The listing builds one solid part. Answer for the finished solid, in the listing's coordinates (mm). Give positions to 0.01 mm unless a question says otherwise; leave off trailing zeros. Order: outer loops, then holes, each group sorted by start corner. A loop starts at its lowest first (then second) coordinate and runs counter-clockwise, first axis right, second up. Notation, with made-up numbers: (89, 63) -> (114, 63) arc R23 cw to (114, 101) -> close; hole circle Ø4 at (27, 68.5). An arc over 180 degrees is marked (long way). Answer as a JSON object with one key per item and string values. Group by question number.
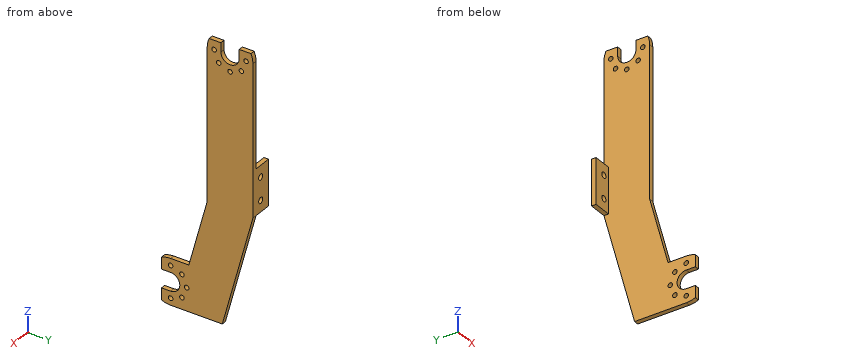
Autodesk Inventor part; units mm, degrees
ref_plane "YZ Plane" through (0, 0, 0) normal (1, 0, 0) x (0, 1, 0)
ref_plane "XZ Plane" through (0, 0, 0) normal (0, 1, 0) x (-1, 0, 0)
ref_plane "XY Plane" through (0, 0, 0) normal (0, 0, 1) x (1, 0, 0)
sketch "スケッチ1" plane through (0, 0, 0) normal (1, 0, 0) x (0, 1, 0)
  line L0 (-20, 60) -> (20, 60)
  line L1 (20, 60) -> (20, -60)
  line L2 (20, -60) -> (-20, -60)
  line L3 (-20, -60) -> (-20, 60)
  point P0 (0, 0)
  dimension "d0" = 120
  dimension "d2" = 40
  dimension "d3" = 20
  dimension "d4" = 60
extrude "押し出し1" add sketch "スケッチ1" along normal blind 2
sketch "スケッチ3" plane through (0, 0, 0) normal (-1, 0, 0) x (0, 0, 1)
  line L0 (60, -20) -> (60, 20)
  line L1 (60, 20) -> (-60, 20)
  line L2 (-60, 20) -> (-60, -20)
  line L3 (-60, -20) -> (60, -20)
  line L4 (-40, -20) -> (-40, -8.0385)
  line L5 (-40, -8.0385) -> (-10, 0)
  line L6 (-10, 0) -> (60, 0)
  line L7 (60, 0) -> (60, 20)
  line L8 (-60, 6.6025) -> (-10, 20)
  point P0 (0, 0)
  dimension "d11" = 20
  dimension "d12" = 15
  dimension "d13" = 15
  dimension "d14" = 20
  dimension "d15" = 120
  dimension "d17" = 70
  dimension "d18" = 70
extrude "押し出し3" cut sketch "スケッチ3" against normal blind 20 contours L6 L5 L4 L3 L2 L8 L1 L0 keep common part
sketch "スケッチ6" plane through (0, 0, 0) normal (-1, 0, 0) x (0, 0, 1)
  line L0 (-40, -8.0385) -> (-40, -20)
  line L1 (-10, 0) -> (-40, -8.0385)
  line L2 (60, 0) -> (-10, 0)
  line L3 (60, 0) -> (60, 20)
  line L4 (60, 20) -> (-10, 20)
  line L5 (-60, 6.6025) -> (-10, 20)
  line L6 (-60, 6.6025) -> (-60, -20)
  line L7 (-60, -20) -> (-40, -20)
  arc A0 (-46, -16) -> (-54, -16) centre (-50, -16) ccw
  arc A1 (56, 14) -> (56, 6) centre (56, 10) ccw
  line L8 (-54, -16) -> (-54, -20)
  line L9 (-46, -16) -> (-46, -20)
  line L10 (56, 14) -> (60, 14)
  line L11 (56, 6) -> (60, 6)
  arc A2 (-40.8348, -20) -> (-40, -16) centre (-50, -16) ccw
  arc A3 (-60, -16) -> (-59.1652, -20) centre (-50, -16) ccw
  arc A4 (56, 0) -> (60, 0.8348) centre (56, 10) ccw
  arc A5 (60, 19.1652) -> (56, 20) centre (56, 10) ccw
  point P0 (0, 0)
  dimension "d39" = 8
  dimension "d40" = 4
  dimension "d41" = 4
  dimension "d42" = 10
  dimension "d43" = 10
extrude "押し出し6" cut sketch "スケッチ6" against normal blind 11 contours L0 A2 L7 L9 A0 L8 A3 L6 L5 L4 A5 L3 L10 A1 L11 A4 L2 L1 keep common part
sketch "スケッチ7" plane through (0, 0, 0) normal (-1, 0, 0) x (0, 0, 1)
  arc A0 (60, 19.1652) -> (56, 20) centre (56, 10) ccw
  arc A1 (-60, -16) -> (-59.1652, -20) centre (-50, -16) ccw
  line L0 (-59.1652, -20) -> (-54, -20)
  line L1 (60, 0.8348) -> (60, 6)
  circle A2 centre (56, 3) radius 1
  circle A3 centre (-57, -16) radius 1
  point P0 (0, 0)
  dimension "d46" = 2
  dimension "d48" = 7
  dimension "d49" = 4
  dimension "d50" = 4
  dimension "d51" = 7
hole "穴1" at (0, -16, -57) at (0, 3, 56) direction (1, 0, 0) diameter 2 end through all
pattern_circular "円形状パターン1" count 5 over 180 about axis through (0, -16, -50) along (1, 0, 0) of "穴1"
pattern_circular "円形状パターン2" count 5 over 180 about axis through (0, 10, 56) along (1, 0, 0) of "穴1"
sketch "スケッチ9" plane through (0, 0, 0) normal (-1, 0, 0) x (0, 0, 1)
  line L0 (56, 20) -> (-10, 20)
  line L1 (60, 14) -> (60, 19.1652)
  line L2 (10, 20) -> (-10, 20)
  line L3 (-10, 20) -> (-10, 18)
  line L4 (-10, 18) -> (10, 18)
  line L5 (10, 18) -> (10, 20)
  point P0 (0, 0)
  dimension "d85" = 2
  dimension "d87" = 20
  dimension "d88" = 50
extrude "押し出し8" add sketch "スケッチ9" along normal blind 8
sketch "スケッチ10" plane through (0, 20, 56) normal (0, 1, 0) x (1, 0, 0)
  line L0 (0, 66) -> (-8, 66)
  line L1 (-8, 46) -> (-8, 66)
  circle A0 centre (-3, 51) radius 1
  circle A1 centre (-3, 61) radius 1
  point P0 (0, 56)
  dimension "d94" = 5
  dimension "d95" = 5
  dimension "d96" = 10
  dimension "d97" = 5
  dimension "d98" = 2
hole "穴3" at (-3, 20, 5) at (-3, 20, -5) direction (0, -1, 0) diameter 2.6 end through all
thread "ねじ5"
thread "ねじ6"
properties part number "10"
(1) A cutting plane is placed at B-B (x = -6.5). Determine the outline of the cut face in (y, z).
(2) A cutting plane is placed at C-C (y = -2.5). Determine the outline of the cut face in (x, z), and give its area (3 significant figures).
(3) A cutting plane is placed at A-A (z = 5). Determine the outline of the cut face in (x, y).
(4) Find the intervals of material crossed by line 1 along Z through (x, y) = (-3, 18.85); line 2 along Z through (x, y) = (1.35, 3); line 3 along X through (y, z) = (19.15, -5), in increasing order. Write a range as [from, to].
(5) Flat-ended cylindrical pins translate along their axes: pin 1 Ø4 at (x, z) = (-3, 5) entering from -Y; pin 2 Ø8 at (y, z) = (15, -15) entering from -X; pin 3 Ø2 at (x, y) = (1, -17.5) entering from +Z. Find the tip coordinate at first contact, or state that the pin passes through.
Check sheet entries:
{
 "1": {"outline": "(18, -10) -> (20, -10) -> (20, 10) -> (18, 10) -> close"},
 "2": {"outline": "(0, -60) -> (2, -60) -> (2, -19.33) -> (0, -19.33) -> close", "area": "81.3 mm2"},
 "3": {"outline": "(-8, 18) -> (-4.3, 18) -> (-4.3, 20) -> (-8, 20) -> close; (-1.7, 18) -> (0, 18) -> (0, 0) -> (2, 0) -> (2, 20) -> (-1.7, 20) -> close"},
 "4": {"line 1": "z = [-10, -6.3], [-3.7, 3.7], [6.3, 10]", "line 2": "z = [-60, 55], [57, 60]", "line 3": "x = [-8, -4.3], [-1.7, 2]"},
 "5": {"pin 1": "stops at y = 18", "pin 2": "stops at x = 0", "pin 3": "stops at z = -40.01"}
}
